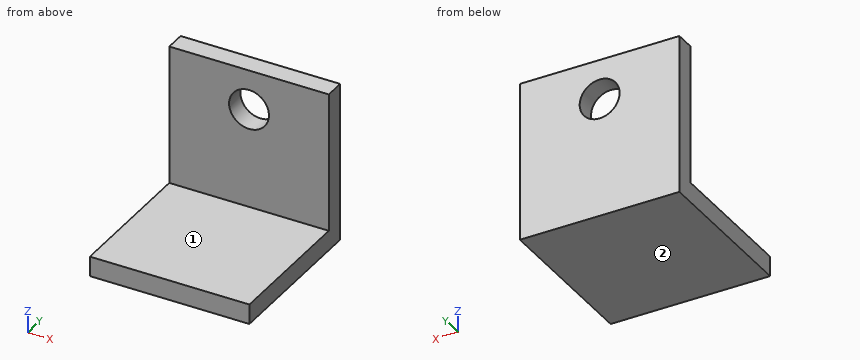
```python
from build123d import *

# Parameters (mm, degrees)
F1_DEPTH = 25.4
F3_D     = 12.7


with BuildPart() as f1:
    # F0 (on Right) → F1 (new body, symmetric)
    with BuildSketch(Plane.YZ):
        Polygon((-50.8, 6.35), (-50.8, 0), (0, 0), (0, 50.8), (-6.35, 50.8), (-6.35, 6.35), align=None)
    extrude(amount=F1_DEPTH, both=True)

    # F3 (through all)
    with Locations(Plane.XZ.offset(6.35)):
        with Locations((0, 38.1)):
            Hole(F3_D / 2)


solid = f1.part
```
CAD build for the part. Positions are in the model's coordinates, mm. Face numbers are marked on the shaded views. A direction names the side the tool comes from. Coordinates: 2 decimals unless noted, no trailing zeros. Write each loop counter-clockwise with the first axis right and the second up, starting at its lowest first coordinate (ties: lowest second). Pieces come first, ordered by that corner, then holes. Notation, with made-up numbers: (38, 35.25) -> (95, 35.25) arc R30 cw to (95, 71.25) -> close; hole circle Ø10 at (-6, 69.25). An arc over 180 degrees is marked (long way). Use CSV: the item, a comma, the result in double quotes. Start each with the question number.
Item 1: Drop flat-ended pins along their axis: P1, Ø11.5, axis at x = 0, z = 38.1, coming from the +Y side; P2, Ø3, axis at x = -18, y = -22, coming from the +Z side; P3, Ø13.5, axis at x = 4.5, z = 21, coming from the -Y side. Give the stop position or say it passes through.
Item 2: Band-saw the part on C-C, the plane x = 16.5. Write the cut outline in (y, z).
Item 3: Band-saw the part on B-B, the plane z = 38.1. Write the cut outline in (x, y), plus the area to 3 significant figures.
Item 4: Wall check: probe 1 along Z at (x, y) = (0, -5); probe 2 along X at (y, z) = (-2, 38); probe 3 along Z at (x, y) = (-13, -35.5). Give the ranges that are in metal, low to high.
Item 5: Band-saw the part on D-D, the plane y = -23. Write the cut outline in (x, z).
Item 6: Tool access for the marked faces 1 and 2: list every direction of +Z, -Z, +X, -X, +Y, -Y with a clear straight run to the whole face (end or side of a thin tool).
Item 7: Band-saw the part on A-A, the plane x = 0. Write the cut outline in (y, z).
Response values:
1,P1,"passes through"
1,P2,"stops at z = 6.35"
1,P3,"stops at y = -6.35"
2,outline,"(-50.8, 0) -> (0, 0) -> (0, 50.8) -> (-6.35, 50.8) -> (-6.35, 6.35) -> (-50.8, 6.35) -> close"
3,outline,"(-25.4, -6.35) -> (-6.35, -6.35) -> (-6.35, 0) -> (-25.4, 0) -> close; (6.35, -6.35) -> (25.4, -6.35) -> (25.4, 0) -> (6.35, 0) -> close"
3,area,"242 mm2"
4,probe 1,"z = 0 to 31.75, 44.45 to 50.8"
4,probe 2,"x = -25.4 to -6.35, 6.35 to 25.4"
4,probe 3,"z = 0 to 6.35"
5,outline,"(-25.4, 0) -> (25.4, 0) -> (25.4, 6.35) -> (-25.4, 6.35) -> close"
6,face 1,"+Z, +X, -X, -Y"
6,face 2,"-Z, +X, -X, +Y, -Y"
7,outline,"(-50.8, 0) -> (0, 0) -> (0, 31.75) -> (-6.35, 31.75) -> (-6.35, 6.35) -> (-50.8, 6.35) -> close; (-6.35, 44.45) -> (0, 44.45) -> (0, 50.8) -> (-6.35, 50.8) -> close"
